CAD build for the part. Positions are in the model's coordinates, mm. A direction names the side the tool comes from. Give positions to 0.01 mm unless a question says otherwise; leave off trailing zeros. Order: outer loops, then holes, each group sorted by start corner. A loop starts at its lowest first (then second) coordinate and runs counter-clockwise, first axis right, second up. Notation, with made-up numbers: (62.5, 59.25) -> (77.5, 59.25) arc R18 ccw to (77.5, 81.25) -> close; hole circle Ø11 at (30.25, 17). An arc over 180 degrees is marked (long way). Answer as CSV lines item,"result".
Autodesk Inventor part; units mm, degrees
ref_plane "YZ Plane" through (0, 0, 0) normal (1, 0, 0) x (0, 1, 0)
ref_plane "XZ Plane" through (0, 0, 0) normal (0, 1, 0) x (-1, 0, 0)
ref_plane "XY Plane" through (0, 0, 0) normal (0, 0, 1) x (1, 0, 0)
sketch "Sketch1" plane through (0, 0, 0) normal (0, 1, 0) x (-1, 0, 0)
  line L0 (0, 0) -> (64, 0)
  line L1 (64, 0) -> (64, -100)
  line L2 (64, -100) -> (0, -100)
  line L3 (0, -100) -> (0, 0)
  dimension "d0" = 64
  dimension "d1" = 100
extrude "Extrusion1" add sketch "Sketch1" along normal blind 1.8
fillet "Fillet1" radius 4 4 edges at (-64, 0.9, 0) (0, 0.9, 0) (0, 0.9, -100) (-64, 0.9, -100)
sketch "Sketch2" plane through (0, 0, 0) normal (0, -1, 0) x (1, 0, 0)
  arc A0 (-64, -96) -> (-60, -100) centre (-60, -96) ccw
  arc A1 (-4, -100) -> (0, -96) centre (-4, -96) ccw
  arc A2 (0, -4) -> (-4, 0) centre (-4, -4) ccw
  arc A3 (-60, 0) -> (-64, -4) centre (-60, -4) ccw
  line L0 (-64, -4) -> (-64, -96)
  line L1 (-60, -100) -> (-60, -96)
  line L2 (-60, -96) -> (-64, -96)
  line L3 (0, -96) -> (-4, -96)
  line L4 (-4, -96) -> (-4, -100)
  line L5 (0, -4) -> (-4, -4)
  line L6 (-4, -4) -> (-4, 0)
  line L7 (-60, 0) -> (-60, -4)
  line L8 (-60, -4) -> (-64, -4)
  point P0 (0, 0)
  point P1 (-60.8, -96.8)
  point P2 (-3.2, -96.8)
  point P3 (-3.2, -3.2)
  point P4 (-60.8, -3.2)
  dimension "d5" = 4
  dimension "d6" = 0.8
  dimension "d7" = 0.8
  dimension "d8" = 0.8
  dimension "d9" = 0.8
  dimension "d10" = 0.8
  dimension "d11" = 0.8
  dimension "d12" = 0.8
  dimension "d13" = 0.8
hole "Hole1" at (-60.8, 0, -96.8) at (-3.2, 0, -96.8) at (-3.2, 0, -3.2) at (-60.8, 0, -3.2) direction (0, 1, 0) diameter 3.2 end through all
sketch "Sketch3" plane through (0, 1.8, 0) normal (0, 1, 0) x (1, 0, 0)
  line L0 (-24.0749, 86.9532) -> (-9.798, 86.9532)
  line L1 (-9.798, 86.9532) -> (-9.798, 74.9855)
  line L2 (-9.798, 74.9855) -> (-24.0749, 74.9855)
  line L3 (-24.0749, 74.9855) -> (-24.0749, 86.9532)
  line L4 (-42.004, 76.8088) -> (-36.0181, 76.8088)
  line L5 (-36.0181, 76.8088) -> (-36.0181, 71.0747)
  line L6 (-36.0181, 71.0747) -> (-42.004, 71.0747)
  line L7 (-42.004, 71.0747) -> (-42.004, 76.8088)
  line L8 (-26.0395, 59.4207) -> (-18.9932, 59.4207)
  line L9 (-18.9932, 59.4207) -> (-18.9932, 52.191)
  line L10 (-18.9932, 52.191) -> (-26.0395, 52.191)
  line L11 (-26.0395, 52.191) -> (-26.0395, 59.4207)
  line L12 (-21.1941, 72.0637) -> (-16.9365, 72.0637)
  line L13 (-16.9365, 72.0637) -> (-16.9365, 67.1402)
  line L14 (-16.9365, 67.1402) -> (-21.1941, 67.1402)
  line L15 (-21.1941, 67.1402) -> (-21.1941, 72.0637)
  line L16 (-31.5453, 82.6589) -> (-26.0395, 82.6589)
  line L17 (-26.0395, 82.6589) -> (-26.0395, 77.9216)
  line L18 (-26.0395, 77.9216) -> (-31.5453, 77.9216)
  line L19 (-31.5453, 77.9216) -> (-31.5453, 82.6589)
  line L20 (-27.0702, 92.6857) -> (-6.8232, 92.6857)
  line L21 (-6.8232, 92.6857) -> (-6.8232, 89.4983)
  line L22 (-6.8232, 89.4983) -> (-27.0702, 89.4983)
  line L23 (-27.0702, 89.4983) -> (-27.0702, 92.6857)
  line L24 (-27.0702, 97.7771) -> (-6.9471, 97.7771)
  line L25 (-6.9471, 97.7771) -> (-6.9471, 94.5771)
  line L26 (-6.9471, 94.5771) -> (-27.0702, 94.5771)
  line L27 (-27.0702, 94.5771) -> (-27.0702, 97.7771)
  line L28 (-27.0702, 9.0883) -> (-6.8232, 9.0883)
  line L29 (-6.8232, 9.0883) -> (-6.8232, 11.9431)
  line L30 (-6.8232, 11.9431) -> (-27.0702, 11.9431)
  line L31 (-27.0702, 11.9431) -> (-27.0702, 9.0883)
  line L32 (-28.1635, 5.4758) -> (-8.1648, 5.4758)
  line L33 (-8.1648, 5.4758) -> (-8.1648, 2.1639)
  line L34 (-8.1648, 2.1639) -> (-28.1635, 2.1639)
  line L35 (-28.1635, 2.1639) -> (-28.1635, 5.4758)
  line L36 (-39.5623, 5.4758) -> (-32.7683, 5.4758)
  line L37 (-32.7683, 5.4758) -> (-32.7683, 1.1716)
  line L38 (-32.7683, 1.1716) -> (-39.5623, 1.1716)
  line L39 (-39.5623, 1.1716) -> (-39.5623, 5.4758)
  line L40 (-55.1326, 3.3237) -> (-50.3337, 3.3237)
  line L41 (-50.3337, 3.3237) -> (-50.3337, 0.6285)
  line L42 (-50.3337, 0.6285) -> (-55.1326, 0.6285)
  line L43 (-55.1326, 0.6285) -> (-55.1326, 3.3237)
  line L44 (-47.0326, 0.6285) -> (-42.004, 0.6285)
  line L45 (-42.004, 0.6285) -> (-42.004, 3.3237)
  line L46 (-42.004, 3.3237) -> (-47.0326, 3.3237)
  line L47 (-47.0326, 3.3237) -> (-47.0326, 0.6285)
  line L48 (-55.1326, 96.8) -> (-50.3337, 96.8)
  line L49 (-50.3337, 96.8) -> (-50.3337, 99.4879)
  line L50 (-50.3337, 99.4879) -> (-55.1326, 99.4879)
  line L51 (-55.1326, 99.4879) -> (-55.1326, 96.8)
  point P0 (0, 0)
extrude "Extrusion2" add sketch "Sketch3" along normal blind 1 contours L0 L1 L2 L3 | L4 L5 L6 L7 | L8 L9 L10 L11 | L12 L13 L14 L15 | L16 L17 L18 L19 | L32 L33 L34 L35
extrude "Extrusion3" add sketch "Sketch3" along normal blind 3 contours L20 L21 L22 L23 | L24 L25 L26 L27 | L31 L30 L29 L28
extrude "Extrusion4" add sketch "Sketch3" along normal blind 1 contours L40 L41 L42 L43 | L47 L46 L45 L44 | L51 L50 L49 L48
extrude "Extrusion5" add sketch "Sketch3" along normal blind 3 contours L36 L37 L38 L39
sketch "Sketch4" plane through (0, 1.8, 0) normal (0, 1, 0) x (1, 0, 0)
  line L0 (-32.7683, 5.4758) -> (-32.7683, 1.1716)
  line L1 (-32.7683, 1.1716) -> (-39.5623, 1.1716)
  line L2 (-39.5623, 1.1716) -> (-39.5623, 5.4758)
  line L3 (-39.5623, 5.4758) -> (-32.7683, 5.4758)
  line L4 (-50.3337, 3.3237) -> (-50.3337, 0.6285)
  line L5 (-50.3337, 0.6285) -> (-55.1326, 0.6285)
  line L6 (-55.1326, 0.6285) -> (-55.1326, 3.3237)
  line L7 (-55.1326, 3.3237) -> (-50.3337, 3.3237)
  line L8 (-55.1326, 96.8) -> (-55.1326, 99.4879)
  line L9 (-55.1326, 99.4879) -> (-50.3337, 99.4879)
  line L10 (-50.3337, 99.4879) -> (-50.3337, 96.8)
  line L11 (-50.3337, 96.8) -> (-55.1326, 96.8)
  line L12 (-47.0326, 0.6285) -> (-47.0326, 3.3237)
  line L13 (-47.0326, 3.3237) -> (-42.004, 3.3237)
  line L14 (-42.004, 3.3237) -> (-42.004, 0.6285)
  line L15 (-42.004, 0.6285) -> (-47.0326, 0.6285)
  line L16 (-6.9471, 97.7771) -> (-6.9471, 94.5771)
  line L17 (-6.9471, 94.5771) -> (-27.0702, 94.5771)
  line L18 (-27.0702, 94.5771) -> (-27.0702, 97.7771)
  line L19 (-27.0702, 97.7771) -> (-6.9471, 97.7771)
  line L20 (-27.0702, 9.0883) -> (-27.0702, 11.9431)
  line L21 (-27.0702, 11.9431) -> (-6.8232, 11.9431)
  line L22 (-6.8232, 11.9431) -> (-6.8232, 9.0883)
  line L23 (-6.8232, 9.0883) -> (-27.0702, 9.0883)
  line L24 (-6.8232, 92.6857) -> (-6.8232, 89.4983)
  line L25 (-6.8232, 89.4983) -> (-27.0702, 89.4983)
  line L26 (-27.0702, 89.4983) -> (-27.0702, 92.6857)
  line L27 (-27.0702, 92.6857) -> (-6.8232, 92.6857)
  line L28 (-8.1648, 5.4758) -> (-8.1648, 2.1639)
  line L29 (-8.1648, 2.1639) -> (-28.1635, 2.1639)
  line L30 (-28.1635, 2.1639) -> (-28.1635, 5.4758)
  line L31 (-28.1635, 5.4758) -> (-8.1648, 5.4758)
  line L32 (-36.0181, 76.8088) -> (-36.0181, 71.0747)
  line L33 (-36.0181, 71.0747) -> (-42.004, 71.0747)
  line L34 (-42.004, 71.0747) -> (-42.004, 76.8088)
  line L35 (-42.004, 76.8088) -> (-36.0181, 76.8088)
  line L36 (-16.9365, 72.0637) -> (-16.9365, 67.1402)
  line L37 (-16.9365, 67.1402) -> (-21.1941, 67.1402)
  line L38 (-21.1941, 67.1402) -> (-21.1941, 72.0637)
  line L39 (-21.1941, 72.0637) -> (-16.9365, 72.0637)
  line L40 (-26.0395, 82.6589) -> (-26.0395, 77.9216)
  line L41 (-26.0395, 77.9216) -> (-31.5453, 77.9216)
  line L42 (-31.5453, 77.9216) -> (-31.5453, 82.6589)
  line L43 (-31.5453, 82.6589) -> (-26.0395, 82.6589)
  line L44 (-18.9932, 59.4207) -> (-18.9932, 52.191)
  line L45 (-18.9932, 52.191) -> (-26.0395, 52.191)
  line L46 (-26.0395, 52.191) -> (-26.0395, 59.4207)
  line L47 (-26.0395, 59.4207) -> (-18.9932, 59.4207)
  line L48 (-9.798, 86.9532) -> (-9.798, 74.9855)
  line L49 (-9.798, 74.9855) -> (-24.0749, 74.9855)
  line L50 (-24.0749, 74.9855) -> (-24.0749, 86.9532)
  line L51 (-24.0749, 86.9532) -> (-9.798, 86.9532)
  circle A0 centre (-3.2, 3.2) radius 1.6
  circle A1 centre (-60.8, 96.8) radius 1.6
  circle A2 centre (-3.2, 96.8) radius 1.6
  circle A3 centre (-60.8, 3.2) radius 1.6
  arc A4 (-60, 100) -> (-64, 96) centre (-60, 96) ccw
  line L52 (-64, 96) -> (-64, 4)
  arc A5 (-64, 4) -> (-60, 0) centre (-60, 4) ccw
  line L53 (-60, 0) -> (-4, 0)
  arc A6 (-4, 0) -> (0, 4) centre (-4, 4) ccw
  line L54 (0, 4) -> (0, 96)
  arc A7 (0, 96) -> (-4, 100) centre (-4, 96) ccw
  line L55 (-4, 100) -> (-60, 100)
  point P0 (0, 0)
sketch "Sketch5" plane through (0, 1.8, 0) normal (0, 1, 0) x (1, 0, 0)
  line L0 (-51.5216, 14.0163) -> (-8.0501, 14.0163)
  line L1 (-8.0501, 14.0163) -> (-8.0501, 50.2303)
  line L2 (-8.0501, 50.2303) -> (-51.5216, 50.2303)
  line L3 (-51.5216, 50.2303) -> (-51.5216, 14.0163)
  line L4 (-51.5216, 50.2303) -> (-45.958, 50.2303)
  line L5 (-45.958, 50.2303) -> (-45.958, 45.2733)
  line L6 (-45.958, 45.2733) -> (-51.5216, 45.2733)
  line L7 (-51.5216, 45.2733) -> (-51.5216, 50.2303)
  circle A0 centre (-48.6054, 11.1502) radius 2.866
  line L8 (-51.5216, 14.0163) -> (-51.471, 11.1006)
  arc A1 (-43.4561, 14.0163) -> (-45.7398, 11.1006) centre (-43.2203, 11.4794) ccw
  circle A2 centre (-10.5958, 52.7257) radius 2.4954
  line L9 (-8.0501, 50.2303) -> (-8.1009, 52.7756)
  arc A3 (-16.0357, 50.2303) -> (-13.0911, 52.7088) centre (-16.6158, 53.908) ccw
  point P0 (0, 0)
extrude "Extrusion6" add sketch "Sketch5" along normal blind 8 contours L0 L3 L6 L5 L2 L1 | A1 A0 L0 | A0 L8 L0 | A0 A1 | L2 A2 L9 | L2 A3 A2 | A2 picked at (-49.5355, 10.9245)
sketch "Sketch7" plane through (0, 0, 0) normal (0, -1, 0) x (1, 0, 0)
  line L0 (-41.7523, -3.2) -> (-19.972, -3.2)
  line L1 (-19.972, -3.2) -> (-19.972, -11.1201)
  line L2 (-19.972, -11.1201) -> (-41.7523, -11.1201)
  line L3 (-41.7523, -11.1201) -> (-41.7523, -3.2)
  point P0 (0, 0)
extrude "Extrusion7" add sketch "Sketch7" along normal blind 3
sketch "Sketch8" plane through (0, 0, 0) normal (0, -1, 0) x (1, 0, 0)
  circle A0 centre (-30.8621, -86.2682) radius 2.9892
  point P0 (0, 0)
extrude "Extrusion8" add sketch "Sketch8" along normal blind 2
sketch "Sketch9" plane through (-30.8621, -2, -86.2682) normal (0, -1, 0) x (1, 0, 0)
  circle A0 centre (0, 0) radius 2.9892
  point P0 (30.8621, 86.2682)
hole "Hole2" at (-30.8621, -2, -86.2682) direction (0, 1, 0) diameter 3.2 end through all
sketch "Sketch10" plane through (0, 1.8, 0) normal (0, 1, 0) x (1, 0, 0)
  line L0 (0, 4) -> (0, 96)
  line L1 (0, 73.518) -> (-14.2183, 73.518)
  line L2 (-14.2183, 73.518) -> (-14.2183, 58.9192)
  line L3 (-14.2183, 58.9192) -> (0, 58.9192)
  line L4 (0, 58.9192) -> (0, 73.518)
  point P0 (0, 0)
extrude "Extrusion9" add sketch "Sketch10" along normal blind 1
properties part number "nanopc_t4"
1) Wall check: line 1 along Z through (x, y) = (-31, 1); line 2 along Z through (x, y) = (-3.2, 1.15); line 3 along X through (y, z) = (0.7, -96.8). Give the ranges that are in metal, low to high. Write a range as [from, to].
Data:
line 1,"z = [-100, -87.86], [-84.67, 0]"
line 2,"z = [-99.92, -98.4], [-95.2, -4.8], [-1.6, -0.08]"
line 3,"x = [-63.92, -62.4], [-59.2, -4.8], [-1.6, -0.08]"
2) Pin check, flat tips, straight feed: P1, Ø2.5, axis at y = 3, z = -10.5, coming from the +X side; P2, Ø5, axis at x = -36, z = -78.5, coming from the -Y side; P3, Ø0.8, axis at x = -44.5, y = 2.5, coming from the +Z side; P4, Ø4, axis at x = -30.86, z = -86.27, coming from the -Y side. Stop position of each tip, or through.
Data:
P1,"stops at x = 0"
P2,"stops at y = 0"
P3,"stops at z = -0.63"
P4,"stops at y = -2"
3) Which spindle directions (+Z, -Z, +X, -X, +Y, -Y) get a long thin tool onto all of the face, cutting with end or side? Do faces 1 (the flat face through (-45, 2.8, -2)), 2 (the flat face through (-31, 6, -50.23)), 3 (the flat face through (-18, 2.8, -4)), 4 (the cylindrical face through (-28.011, -0.986, -87.166)), 5 (the flat face through (-30, -2, -88)). Say none if no direction does.
Data:
face 1,"+Z, -X, +Y"
face 2,"-X, +Y"
face 3,"+Z, +X, +Y"
face 4,"-Y"
face 5,"-Z, +X, -X, -Y"
4) Pull direction X, two halves, no side cores. Call faces 6 (the flat face through (-32.768, 3, -3)), 7 (the flat face through (-6.823, 3, -91)), 8 (the flat face through (-53, 2.8, -2)): pulls with the +X half, pulls with the -X half, needs draft (parallel to the pull), parting line crosses it, or undercut.
Data:
face 6,"undercut"
face 7,"pulls with the +X half"
face 8,"needs draft"
5) Band-saw the part on B-B, the plane y = -1. Write the cut outline in (x, z).
Data:
outline,"(-41.75, -11.12) -> (-19.97, -11.12) -> (-19.97, -3.2) -> (-41.75, -3.2) -> close; circle Ø5.98 at (-30.86, -86.27); hole circle Ø3.2 at (-30.86, -86.27)"
6) Band-saw the part on A-A, the plane z = -39.5. Write the cut outline in (x, y).
Data:
outline,"(-64, 0) -> (0, 0) -> (0, 1.8) -> (-8.05, 1.8) -> (-8.05, 9.8) -> (-51.52, 9.8) -> (-51.52, 1.8) -> (-64, 1.8) -> close"
7) Band-saw the part on C-C, the plane y = 6.75. Write the cut outline in (x, z), then the cut area to 3 significant figures.
Data:
outline,"(-51.52, -45.27) -> (-45.96, -45.27) -> (-45.96, -50.23) -> (-16.04, -50.23) arc R3.72 cw to (-13.09, -52.71) arc R2.5 ccw (long way) to (-8.1, -52.73) -> (-8.05, -50.23) -> (-8.05, -14.02) -> (-43.46, -14.02) arc R2.55 cw to (-45.74, -11.1) arc R2.87 ccw to (-51.47, -11.1) -> (-51.52, -14.02) -> close"
area,"1,600 mm2"
